Work out the finished part from the listing and answer in its coordinate system (mm). Face numbers are marked on the shaded views. A direction names the side the tool comes from. Coordinates: 2 decimals unless noted, no trailing zeros. Order: outer loops, then holes, each group sorted by start corner. A loop starts at its lowest first (then second) coordinate and runs counter-clockwise, first axis right, second up. Notation, with made-up numbers: (2, 0.25) -> (38, 0.25) arc R13 cw to (38, 25.25) -> close; hole circle Ø7 at (32, -26.5). An arc over 180 degrees is marked (long way). Use one line per item in the form item = value.
from build123d import *

# Parameters (mm, degrees)
CROQUIS1_W              = 110
CROQUIS1_H              = 50.8
SALIENTE_EXTRUIR1_DEPTH = 12.7
CROQUIS2_W              = 50.8
CROQUIS2_H              = 220
SALIENTE_EXTRUIR2_DEPTH = 12.7
CROQUIS4_W              = 25.4
CROQUIS4_H              = 12.7
SALIENTE_EXTRUIR3_DEPTH = 57.3
CROQUIS5_W              = 50.8
CROQUIS5_H              = 50.8
CROQUIS5_W_2            = 59.2
CORTAR_EXTRUIR1_DEPTH   = 211.184323868


with BuildPart() as part:
    # Croquis1 → Saliente-Extruir1 (new body)
    with BuildSketch(Plane.XY):
        Rectangle(CROQUIS1_W, CROQUIS1_H)
    extrude(amount=SALIENTE_EXTRUIR1_DEPTH)

    # Croquis2 → Saliente-Extruir2 (add)
    with BuildSketch(Plane(origin=(0, 0, 0), x_dir=(-1, 0, 0), z_dir=(0, 0, -1))):
        with Locations((-29.6, 84.6)):
            Rectangle(CROQUIS2_W, CROQUIS2_H)
    extrude(amount=SALIENTE_EXTRUIR2_DEPTH)

    # Croquis4 → Saliente-Extruir3 (add)
    with BuildSketch(Plane(origin=(0, 0, -12.7), x_dir=(-1, 0, 0), z_dir=(0, 0, -1))):
        Polygon((-42.3, 194.6), (-55, 194.6), (-55, 143.8), (-42.3, 143.8), (-42.3, 181.9), align=None)
        with Locations((-29.6, 188.25)):
            Rectangle(CROQUIS4_W, CROQUIS4_H)
    extrude(amount=SALIENTE_EXTRUIR3_DEPTH)

    # Croquis5 → Cortar-Extruir1 (cut, through all)
    with BuildSketch(Plane(origin=(0, 0, -12.7), x_dir=(-1, 0, 0), z_dir=(0, 0, -1))):
        Polygon((-55, 143.8), (-55, 25.4), (-4.2, 25.4), (-4.2, 194.6), (-16.9, 194.6), (-16.9, 181.9), (-42.3, 181.9), (-42.3, 143.8), align=None)
        with Locations((-29.6, 0)):
            Rectangle(CROQUIS5_W, CROQUIS5_H)
        with Locations((25.4, 0)):
            Rectangle(CROQUIS5_W_2, CROQUIS5_H)
    extrude(amount=-CORTAR_EXTRUIR1_DEPTH, mode=Mode.SUBTRACT)


solid = part.part
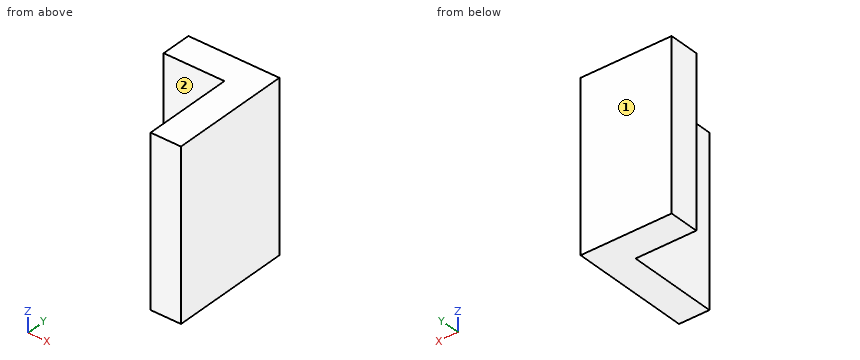
(1) Section B-B on x = 33 is taken. Write down the section's boundary in (y, z).
Data:
outline = (181.9, -70) -> (194.6, -70) -> (194.6, 0) -> (181.9, 0) -> close
(2) Section A-A on z = -29 is taken. Write down the section's boundary in (x, y).
Data:
outline = (16.9, 181.9) -> (42.3, 181.9) -> (42.3, 143.8) -> (55, 143.8) -> (55, 194.6) -> (16.9, 194.6) -> close
(3) Each of these flat-tipped pins is pushed along its axis until it touches: P1, Ø12, axis at y = 159.5, z = -28.5, coming from the -X side; P2, Ø8, axis at x = 42, z = -55.5, coming from the -Y side; P3, Ø7.5, axis at x = 34.5, z = -22, coming from the -Y side. Where does it stop, or does it pass through?
Data:
P1 = 42.3
P2 = 143.8
P3 = 181.9
(4) Which of the six approach directions +Z, -Z, +X, -X, +Y, -Y give full straight-line access (tool end or side, diameter ignored) to the marked faces 1 and 2?
Data:
face_1 = +Z, -Z, +X, -X, +Y
face_2 = +Z, -Z, -X, -Y
(5) Section C-C on y = 152 is taken. Write down the section's boundary in (x, z), plus the area to 3 significant figures.
Data:
outline = (42.3, -70) -> (55, -70) -> (55, 0) -> (42.3, 0) -> close
area = 889 mm²
(6) Straight lines are drawn through the part: line 1 along X through (y, z) = (161.5, -20); line 2 along Y through (x, z) = (27, -20). For each, find the intervals that lie inside material, in ascending order.
Data:
line_1 = 42.3 to 55
line_2 = 181.9 to 194.6
